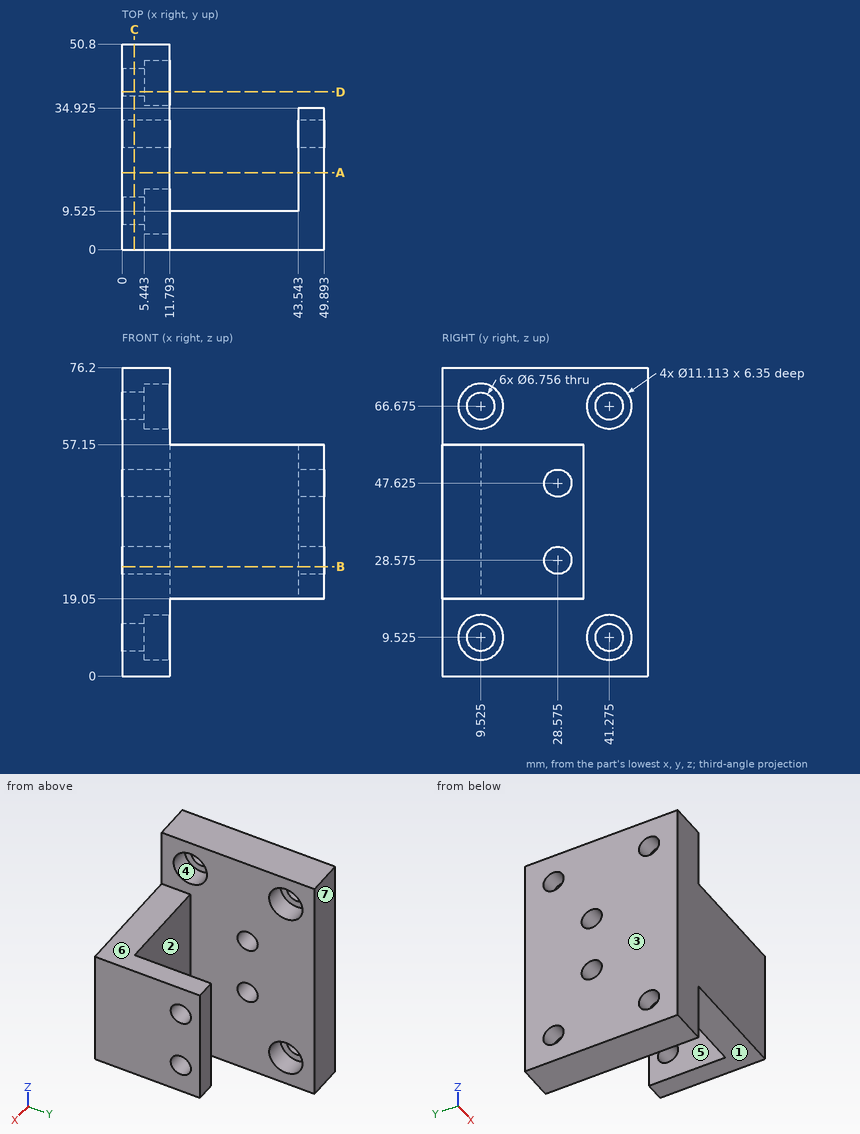
The drawing under review shows one solid part. Ordinate dimensions are in mm from its lowest x, y, z. A direction names the side the tool comes from. Coordinates: 2 decimals unless noted, no trailing zeros. Write each loop counter-clockwise with the first axis right and the second up, starting at its lowest first coordinate (ties: lowest second). Pieces come first, ordered by that corner, then holes. Notation, with made-up numbers: (5.25, -23) -> (39.25, -23) arc R12 ccw to (39.25, -11) -> close; hole circle Ø6 at (89.25, 7.25). An arc over 180 degrees is marked (long way). Write each question's results on one line, items separated by ' | '. Start each with the question number.
1) Consider section A-A (y = 19). Write out the cut boundary in (x, z), plus the area to 3 significant figures.
2) Consider section D-D (y = 39). Write out the cut boundary in (x, z) (1 decimal).
3) The part is to be moulded in two halves that separate along X. For the marked faces 1, 2 and 3, say which applies: +X half, -X half, draft (parallel to the pull), parting line (faces both ways), or undercut.
4) Insertion check: pin 1 (5 mm diameter, centred on x = 42, z = 20.5, fed in from +Y) (1 decimal); pin 2 (3.5 mm diameter, centred on y = 7, z = 10.5, fed in from +X); pin 3 (17.5 mm diameter, centred on x = 37.5, y = 22.5, fed in from +Z); pin 4 (4 mm diameter, centred on y = 28.575, z = 47.625, fed in from -X). Each pin has a flat end and moves straight along its axis. Give the tip position at first contact, or say it passes through.
5) Consider section C-C (x = 3). Write out the cut boundary in (y, z) (1 decimal).
6) Consider section B-B (z = 27). Write out the cut boundary in (x, y) (1 decimal).
7) Wall thickness on L1, parallel to X at y = 34, z = 37.5; L2, parallel to X at y = 43, z = 22.5; L3, parallel to Y at x = 15.5, z = 42 (1 decimal): over which ranges is each line inside the solid? List them lowest first. Write a range as [from, to].
8) For the marked faces 4, 5, 6 and 7, list the 3-axis set-ups (+Z, -Z, +X, -X, +Y, -Y) from which the entire face can be reached by the end or side of a thin tool; tool diameter is ignored.
Geometry says:
1) outline: (0, 0) -> (11.79, 0) -> (11.79, 76.2) -> (0, 76.2) -> close; (43.54, 19.05) -> (49.89, 19.05) -> (49.89, 57.15) -> (43.54, 57.15) -> close | area: 1,140 mm^2
2) outline: (0, 0) -> (11.8, 0) -> (11.8, 4.5) -> (5.4, 4.5) -> (5.4, 7) -> (0, 7) -> close; (0, 12) -> (5.4, 12) -> (5.4, 14.6) -> (11.8, 14.6) -> (11.8, 61.6) -> (5.4, 61.6) -> (5.4, 64.2) -> (0, 64.2) -> close; (0, 69.2) -> (5.4, 69.2) -> (5.4, 71.7) -> (11.8, 71.7) -> (11.8, 76.2) -> (0, 76.2) -> close
3) face 1: draft | face 2: undercut | face 3: -X half
4) pin 1: y = 34.9 | pin 2: x = 5.44 | pin 3: z = 57.15 | pin 4: through
5) outline: (0, 0) -> (50.8, 0) -> (50.8, 76.2) -> (0, 76.2) -> close; hole circle Ø6.8 at (9.5, 9.5); hole circle Ø6.8 at (9.5, 66.7); hole circle Ø6.8 at (28.6, 28.6); hole circle Ø6.8 at (28.6, 47.6); hole circle Ø6.8 at (41.3, 9.5); hole circle Ø6.8 at (41.3, 66.7)
6) outline: (0, 0) -> (49.9, 0) -> (49.9, 25.6) -> (43.5, 25.6) -> (43.5, 9.5) -> (11.8, 9.5) -> (11.8, 25.6) -> (0, 25.6) -> close; (0, 31.6) -> (11.8, 31.6) -> (11.8, 50.8) -> (0, 50.8) -> close; (43.5, 31.6) -> (49.9, 31.6) -> (49.9, 34.9) -> (43.5, 34.9) -> close
7) L1: [0, 11.79], [43.54, 49.89] | L2: [0, 11.79] | L3: [0, 9.5]
8) face 4: +X | face 5: +Z, -Z, +Y | face 6: +Z, +X, +Y, -Y | face 7: +Z, -Z, +X, -X, +Y
